Verification items for the finished model (mm, model axes). Give positions to 0.01 mm unless a question says otherwise; leave off trailing zeros. Write each loop counter-clockwise with the first axis right and the second up, starting at its lowest first coordinate (ties: lowest second). Pieces come first, ordered by that corner, then holes. Notation, with made-up numbers: (22.5, 75) -> (41.5, 75) arc R15 ccw to (41.5, 84) -> close; hole circle Ø10 at (80, 89.5). An arc over 180 degrees is marked (long way). Answer as CSV lines item,"result".
```python
from build123d import *

# Parameters (mm, degrees)
F0_R     = 3.5
F0_W     = 205.5
F0_H     = 7.5
F1_DEPTH = 7
F2_R     = 3.5
F2_W     = 205.5
F2_H     = 7.5
F3_DEPTH = 5


# Not quite as in the source:
# - a feature of the source that left no trace in its solid (it failed there, or was rolled back) is left out


with BuildPart() as f1:
    # F0 (on Top) → F1 (new body)
    with BuildSketch(Plane.XY):
        with BuildLine():
            Line((-115.25, 43.0697486343), (-115.25, 28.0697486343))
            ThreePointArc((-115.25, 28.0697486343), (-114.1583269132, 24.4641973588), (-111.25, 22.0697486343))
            Line((-111.25, 22.0697486343), (-111.25, -7.4302513657))
            ThreePointArc((-111.25, -7.4302513657), (-113.3461940777, -18.0264454434), (-102.75, -15.9302513657))
            Line((-102.75, -15.9302513657), (102.75, -15.9302513657))
            ThreePointArc((102.75, -15.9302513657), (113.3461940777, -18.0264454434), (111.25, -7.4302513657))
            Line((111.25, -7.4302513657), (111.25, 22.0697486343))
            ThreePointArc((111.25, 22.0697486343), (114.1583269132, 24.4641973588), (115.25, 28.0697486343))
            Line((115.25, 28.0697486343), (115.25, 43.0697486343))
            Line((115.25, 43.0697486343), (-115.25, 43.0697486343))
        make_face()
        with Locations((-108.75, -13.4302513657)):
            Circle(F0_R, mode=Mode.SUBTRACT)
        with Locations((108.75, -13.4302513657)):
            Circle(F0_R, mode=Mode.SUBTRACT)
        with BuildLine():
            Line((-102.75, 25.5697486343), (102.75, 25.5697486343))
            ThreePointArc((102.75, 25.5697486343), (104.1538059223, 23.4735545566), (106.25, 22.0697486343))
            Line((106.25, 22.0697486343), (106.25, -7.4302513657))
            ThreePointArc((106.25, -7.4302513657), (104.1538059223, -8.834057288), (102.75, -10.9302513657))
            Line((102.75, -10.9302513657), (-102.75, -10.9302513657))
            ThreePointArc((-102.75, -10.9302513657), (-104.1538059223, -8.834057288), (-106.25, -7.4302513657))
            Line((-106.25, -7.4302513657), (-106.25, 22.0697486343))
            ThreePointArc((-106.25, 22.0697486343), (-104.1538059223, 23.4735545566), (-102.75, 25.5697486343))
        make_face(mode=Mode.SUBTRACT)
        with Locations((-108.75, 28.0697486343)):
            Circle(F0_R, mode=Mode.SUBTRACT)
        with Locations((0, 34.3197486343)):
            Rectangle(F0_W, F0_H, mode=Mode.SUBTRACT)
        with Locations((108.75, 28.0697486343)):
            Circle(F0_R, mode=Mode.SUBTRACT)
    extrude(amount=F1_DEPTH)

    # F2 (on face) → F3 (join)
    with BuildSketch(Plane.XY.offset(7)):
        with BuildLine():
            Line((115.25, 43.0697486343), (-115.25, 43.0697486343))
            Line((-115.25, 43.0697486343), (-115.25, 28.0697486343))
            ThreePointArc((-115.25, 28.0697486343), (-114.1583269132, 24.4641973588), (-111.25, 22.0697486343))
            ThreePointArc((-111.25, 22.0697486343), (-108.75, 21.5697486343), (-106.25, 22.0697486343))
            ThreePointArc((-106.25, 22.0697486343), (-104.1538059223, 23.4735545566), (-102.75, 25.5697486343))
            Line((-102.75, 25.5697486343), (102.75, 25.5697486343))
            ThreePointArc((102.75, 25.5697486343), (104.1538059223, 23.4735545566), (106.25, 22.0697486343))
            ThreePointArc((106.25, 22.0697486343), (108.75, 21.5697486343), (111.25, 22.0697486343))
            ThreePointArc((111.25, 22.0697486343), (114.1583269132, 24.4641973588), (115.25, 28.0697486343))
            Line((115.25, 28.0697486343), (115.25, 43.0697486343))
        make_face()
        with Locations((-108.75, 28.0697486343)):
            Circle(F2_R, mode=Mode.SUBTRACT)
        with Locations((108.75, 28.0697486343)):
            Circle(F2_R, mode=Mode.SUBTRACT)
        with Locations((0, 34.3197486343)):
            Rectangle(F2_W, F2_H, mode=Mode.SUBTRACT)
    extrude(amount=F3_DEPTH)


solid = f1.part
```
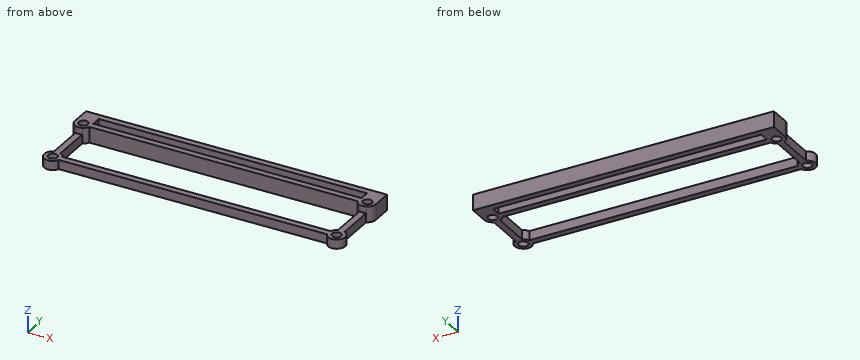
1) Depth check by flat-ended pin: pin 1 (2 mm diameter, centred on y = 3, z = 8.5, fed in from +X); pin 2 (2 mm diameter, centred on y = 10, z = 2.5, fed in from +X); pin 3 (3.5 mm diameter, centred on x = -50, z = 8, fed in from -Y); pin 4 (2 mm diameter, centred on y = 2.5, z = 5, fed in from -X). Enter the tip coordinate at first touch or a pass-through.
Reported:
pin 1,"through"
pin 2,"x = 111.25"
pin 3,"y = -15.93"
pin 4,"x = -111.25"
2) Section check A-A (x = 53). Record the boundary of the cut face in (y, z).
Reported:
outline,"(-15.93, 0) -> (-10.93, 0) -> (-10.93, 7) -> (-15.93, 7) -> close; (25.57, 0) -> (30.57, 0) -> (30.57, 12) -> (25.57, 12) -> close; (38.07, 0) -> (43.07, 0) -> (43.07, 12) -> (38.07, 12) -> close"
3) Section check D-D (x = -108.75). Record the boundary of the cut face in (y, z), and give its area (4 significant figures).
Reported:
outline,"(-19.93, 0) -> (-16.93, 0) -> (-16.93, 7) -> (-19.93, 7) -> close; (-9.93, 0) -> (24.57, 0) -> (24.57, 12) -> (21.57, 12) -> (21.57, 7) -> (-9.93, 7) -> close; (31.57, 0) -> (43.07, 0) -> (43.07, 12) -> (31.57, 12) -> close"
area,"415.5 mm²"
4) Section check C-C (z = 3.5). Record the boundary of the cut face in (x, y).
Reported:
outline,"(-115.25, 28.07) arc R6.5 ccw to (-111.25, 22.07) -> (-111.25, -7.43) arc R6.5 ccw (long way) to (-102.75, -15.93) -> (102.75, -15.93) arc R6.5 ccw (long way) to (111.25, -7.43) -> (111.25, 22.07) arc R6.5 ccw to (115.25, 28.07) -> (115.25, 43.07) -> (-115.25, 43.07) -> close; hole circle Ø7 at (-108.75, -13.43); hole circle Ø7 at (-108.75, 28.07); hole (-106.25, -7.43) arc R6.5 cw to (-102.75, -10.93) -> (102.75, -10.93) arc R6.5 cw to (106.25, -7.43) -> (106.25, 22.07) arc R6.5 cw to (102.75, 25.57) -> (-102.75, 25.57) arc R6.5 cw to (-106.25, 22.07) -> close; hole (-102.75, 30.57) -> (102.75, 30.57) -> (102.75, 38.07) -> (-102.75, 38.07) -> close; hole circle Ø7 at (108.75, -13.43); hole circle Ø7 at (108.75, 28.07)"
5) Section check B-B (y = -0.5). Record the boundary of the cut face in (x, z).
Reported:
outline,"(-111.25, 0) -> (-106.25, 0) -> (-106.25, 7) -> (-111.25, 7) -> close; (106.25, 0) -> (111.25, 0) -> (111.25, 7) -> (106.25, 7) -> close"
6) Scan lines: line 1 along Y through (x, z) = (63, 4.25); line 2 along Y through (x, z) = (-108.75, 2.75); line 3 along Y through (x, z) = (-54, 9.5). Record each from-to range of solid material in increasing order.
Reported:
line 1,"-15.93 to -10.93, 25.57 to 30.57, 38.07 to 43.07"
line 2,"-19.93 to -16.93, -9.93 to 24.57, 31.57 to 43.07"
line 3,"25.57 to 30.57, 38.07 to 43.07"
